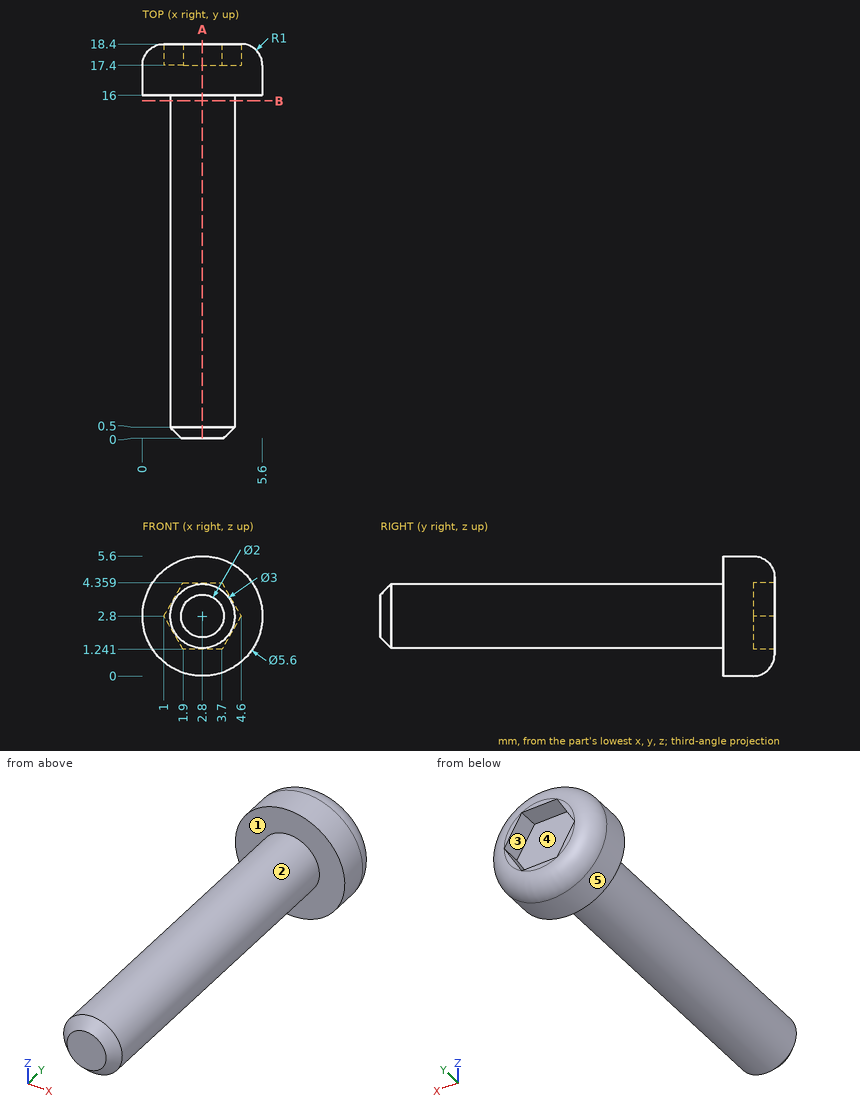
Here's the drawing with two shaded views (mm, measured from the low corner). I have some questions. A direction names the side the tool comes from. Give positions to 0.01 mm unless a question says otherwise; leave off trailing zeros. Loops run counter-clockwise (first coordinate to the right, second up) from the corner with the lowest first, then second, coordinate; pieces in that order, holes last. Notation, with made-up numbers: (-19, -8) -> (14, -8) arc R13 cw to (14, 13) -> close; hole circle Ø11 at (2.5, -3.75). An arc over 180 degrees is marked (long way). Answer as a JSON object with one key per item and string values. Group by question number.
Item 1: Imagine slicing it at B-B on y = 15.75. Write out the boundary of the cut face in (x, z).
Item 2: On a 3-axis mill with a long thin cutter (end or side, diameter ignored), from which of +Z, -Z, +X, -X, +Y, -Y can I reach the whole of each face in a straight line? I mean the marked faces 4 and 5. Say none if no direction works.
Item 3: Will these pins go through, and if not, where does the flat tip stop? pin 1 (3 mm diameter, centred on y = 2, z = 1, fed in from -X); pin 2 (2 mm diameter, centred on y = 9.5, z = 1.5, fed in from +X); pin 3 (1.1 mm diameter, centred on x = 3, y = 18, fed in from -Z).
Item 4: Imagine slicing it at A-A on x = 2.8. Write out the boundary of the cut face in (y, z).
Item 5: I need wall thicknesses on L1, parallel to Z at x = 4, y = 6.5; L2, parallel to Y at x = 3.5, z = 1.2; L3, parallel to X at y = 14.25, z = 2.75. Which ranges of each line are inside material? Lowest first, please.
Item 6: Thinking about a two-plate mould opening in Z: for the marked faces 1, 2 and 3, which applies, pulls with the +Z half, pulls with the -Z half, needs draft (parallel to the pull), parting line crosses it, or undercut?
Answer list:
{
 "1": {"outline": "circle Ø3 at (2.8, 2.8)"},
 "2": {"face 4": "+Y", "face 5": "+Y, -Y"},
 "3": {"pin 1": "stops at x = 1.33", "pin 2": "stops at x = 4.27", "pin 3": "stops at z = 0"},
 "4": {"outline": "(0, 1.8) -> (0.5, 1.3) -> (16, 1.3) -> (16, 0) -> (17.4, 0) arc R1 ccw to (18.4, 1) -> (18.4, 1.24) -> (17.4, 1.24) -> (17.4, 4.36) -> (18.4, 4.36) -> (18.4, 4.6) arc R1 ccw to (17.4, 5.6) -> (16, 5.6) -> (16, 4.3) -> (0.5, 4.3) -> (0, 3.8) -> close"},
 "5": {"L1": "z = 1.9 to 3.7", "L2": "y = 16 to 18.4", "L3": "x = 1.3 to 4.3"},
 "6": {"face 1": "needs draft", "face 2": "parting line crosses it", "face 3": "undercut"}
}
